Geometry: see drawing. Coordinates: mm, zero at the bounding-box minimum. A direction names the side the tool comes from. Round coordinates to 2 decimals unless told otherwise and drop trailing zeros. Order: outer loops, then holes, each group sorted by start corner. A loop starts at its lowest first (then second) coordinate and runs counter-clockwise, first axis right, second up. Notation, with made-up numbers: (23, -36) -> (79, -36) arc R13 ccw to (79, -21) -> close; hole circle Ø3 at (-5, 16). An arc over 180 degrees is marked (long way). Write item = value, one per line. Start each with the question number.
(1) Cut plane C-C on x = 23. Give the number of separate pieces and of enclosed holes in the cut face, then the cut area to 3 significant figures.
(2) Reachability of the marked faces 1 and 2 from +Z, -Z, +X, -X, +Y, -Y: full face, straight path, thin tool, end or side. Return the list, or none.
(3) Cut plane B-B on y = 14. Return the cut outline in (x, z) (1 decimal).
(4) Contact query for flat-ended pins moving along their axis: pin 1 Ø8 at (x, y) = (13.5, 10.5) entering from +Z; pin 2 Ø1.5 at (y, z) = (16.5, 15) entering from +X. Output: stop coordinate, or through.
(5) Draft query along Z for the marked faces 3, 4, 5 and 6. Return one class per face: released by +Z, released by -Z, zero draft, split by the parting line, or undercut.
(6) Cut plane A-A on z = 5. Return the cut outline in (x, y) (1 decimal), then the cut area to 3 significant figures.
(7) Ray query, line 1 (Y direction, x = 16.5, z = 15) (1 decimal); line 2 (Z direction, x = 13, y = 13) (1 decimal); line 3 (Y direction, x = 22.5, z = 29) (1 decimal). Return the intervals inside material, ascending.
(8) Cut plane D-D on z = 24. Return the cut outline in (x, y) (1 decimal).
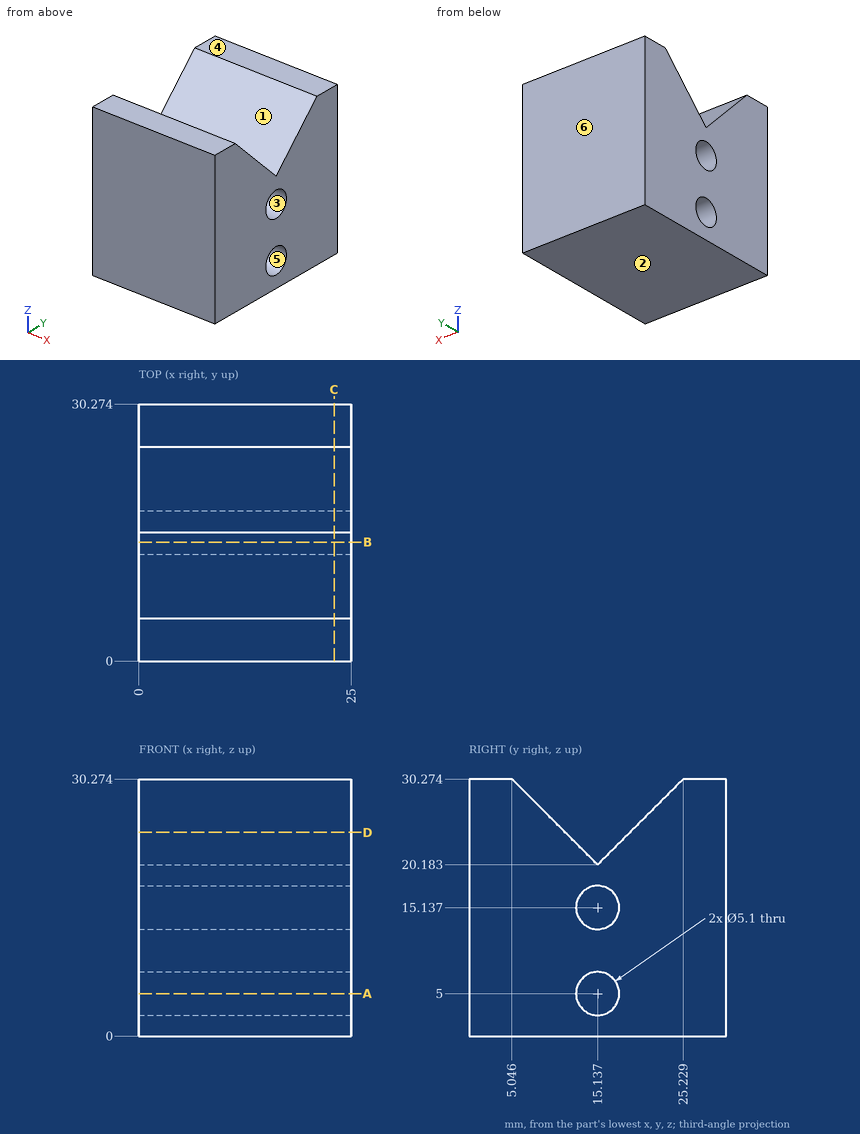
Evaluation:
q1.separate_pieces = 1
q1.enclosed_holes = 2
q1.area = 774 mm^2
q2.face_1 = +Z, +X, -X
q2.face_2 = -Z, +X, -X, +Y, -Y
q3.outline = (0, 0) -> (25, 0) -> (25, 2.7) -> (0, 2.7) -> close; (0, 7.3) -> (25, 7.3) -> (25, 12.9) -> (0, 12.9) -> close; (0, 17.4) -> (25, 17.4) -> (25, 21.3) -> (0, 21.3) -> close
q4.pin_1 = 28.82
q4.pin_2 = through
q5.face_3 = undercut
q5.face_4 = released by +Z
q5.face_5 = undercut
q5.face_6 = zero draft
q6.outline = (0, 0) -> (25, 0) -> (25, 12.6) -> (0, 12.6) -> close; (0, 17.7) -> (25, 17.7) -> (25, 30.3) -> (0, 30.3) -> close
q6.area = 629 mm^2
q7.line_1 = 0 to 12.6, 17.7 to 30.3
q7.line_2 = 0 to 3.6, 6.4 to 13.7, 16.5 to 22.3
q7.line_3 = 0 to 6.3, 24 to 30.3
q8.outline = (0, 0) -> (25, 0) -> (25, 11.3) -> (0, 11.3) -> close; (0, 19) -> (25, 19) -> (25, 30.3) -> (0, 30.3) -> close
